Part model, mm, in its own coordinate system. Face numbers are marked on the shaded views. A direction names the side the tool comes from. Coordinates: 2 decimals unless noted, no trailing zeros. Write each loop counter-clockwise with the first axis right and the second up, starting at its lowest first coordinate (ties: lowest second). Pieces come first, ordered by that corner, then holes. Notation, with made-up numbers: (-9.5, 19.5) - (-1.5, 19.5) arc R21 cw to (-1.5, 47.5) - close; hole circle Ø9 at (-28.5, -31). An arc over 180 degrees is marked (long way). Write each question's results on one line, items separated by ' | '.
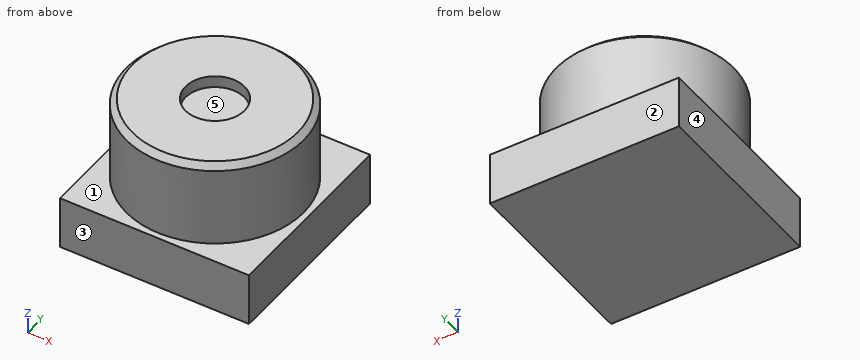
from build123d import *

# Parameters (mm, degrees)
SKETCH005_W     = 8
SKETCH005_H     = 8
PAD003_DEPTH    = 2.25
SKETCH006_R     = 3.75
PAD004_DEPTH    = 3.6
SKETCH007_R     = 1.25
POCKET001_DEPTH = 0.5
CHAMFER001_SIZE = 0.25


with BuildPart() as part:
    # Sketch005 (on Face1 of CopyThickness) → Pad003 (new body)
    with BuildSketch(Plane.XY.offset(3.5)):
        with Locations((0, 12.5)):
            Rectangle(SKETCH005_W, SKETCH005_H)
    extrude(amount=PAD003_DEPTH)

    # Sketch006 (on Face6 of Pad003) → Pad004 (join)
    with BuildSketch(Plane.XY.offset(5.75)):
        with Locations((0, 12.5)):
            Circle(SKETCH006_R)
    extrude(amount=PAD004_DEPTH)

    # Sketch007 (on Face8 of Pad004) → Pocket001 (cut)
    with BuildSketch(Plane.XY.offset(9.35)):
        with Locations((0, 12.5)):
            Circle(SKETCH007_R)
    extrude(amount=-POCKET001_DEPTH, mode=Mode.SUBTRACT)

    # Chamfer001
    chamfer001_edges = [part.edges().sort_by_distance(p)[0] for p in [
        (-3.75, 12.5, 9.35),
    ]]
    chamfer(chamfer001_edges, length=CHAMFER001_SIZE)


solid = part.part
(1) Saw through at A-A on x = 0. Write the cut outline in (y, z), then the cut area to 3 significant figures.
Return value:
outline: (8.5, 3.5) - (16.5, 3.5) - (16.5, 5.75) - (16.25, 5.75) - (16.25, 9.1) - (16, 9.35) - (13.75, 9.35) - (13.75, 8.85) - (11.25, 8.85) - (11.25, 9.35) - (9, 9.35) - (8.75, 9.1) - (8.75, 5.75) - (8.5, 5.75) - close | area: 43.7 mm^2
(2) Saw through at B-B on y = 12.5. Write the cut outline in (x, z), then the cut area to 3 significant figures.
Return value:
outline: (-4, 3.5) - (4, 3.5) - (4, 5.75) - (3.75, 5.75) - (3.75, 9.1) - (3.5, 9.35) - (1.25, 9.35) - (1.25, 8.85) - (-1.25, 8.85) - (-1.25, 9.35) - (-3.5, 9.35) - (-3.75, 9.1) - (-3.75, 5.75) - (-4, 5.75) - close | area: 43.7 mm^2
(3) Flat gauge pins, fed straight in: P1, Ø3, axis at x = 3, z = 7, coming from the +Y side; P2, Ø3, axis at y = 11, z = 8, coming from the -X side; P3, Ø1.2, axis at x = 0, y = 13, coming from the +Z side. Where does each tip first touch, or does it go through?
Return value:
P1: stops at y = 16.5 | P2: stops at x = -3.75 | P3: stops at z = 8.85
(4) 3-axis set-ups, long thin cutter, end or side, ignore diameter. For the marked faces 1 and 2: which of +Z, -Z, +X, -X, +Y, -Y reach the whole face in a straight line?
Return value:
face 1: +Z | face 2: +Z, -Z, +X, -X, +Y
(5) Wall check: line 1 (Y direction, x = 0, z = 9.2); line 2 (Z direction, x = -0.5, y = 12.75); line 3 (Y direction, x = -0.25, z = 6.65). Give the ranges that are in metal, low to high. Write a range as from..to.
Return value:
line 1: y = 8.85..11.25, 13.75..16.15 | line 2: z = 3.5..8.85 | line 3: y = 8.76..16.24
(6) Two-plate mould, pull along X, no slides. Class the marked faces 3, 4 and 5: released by +X, released by -X, zero draft, split by the parting line, or undercut.
Return value:
face 3: zero draft | face 4: released by -X | face 5: undercut
(7) Saw through at C-C on z = 7.95. Write the cut outline in (x, y), then the cut area to 3 significant figures.
Return value:
outline: circle Ø7.5 at (0, 12.5) | area: 44.2 mm^2
